Part model, mm, in its own coordinate system. A direction names the side the tool comes from. Round coordinates to 2 decimals unless told otherwise and drop trailing zeros. Loops run counter-clockwise (first coordinate to the right, second up) from the corner with the lowest first, then second, coordinate; pieces in that order, holes last. Notation, with made-up numbers: M 78,11 L 118,11 A31 ccw 118,49 Z; hole C 36.5,28 d6. An arc over 180 degrees is marked long. Answer as CSV lines item,"result". Start each with the question number.
Item 1: Wall check: line 1 (X direction, y = 2.6, z = -37); line 2 (X direction, y = 1.75, z = -47.5); line 3 (X direction, y = 0.7, z = -57). Give the ranges that are in metal, low to high.
Item 2: Drop a flat-ended pin along its axis: pin 1 Ø1 at (x, y) = (46.5, 2.5) entering from -Z. Give the stop position or say it passes through.
Item 3: Which spindle directions (+Z, -Z, +X, -X, +Y, -Y) get a long thin tool onto all of the face, cutting with end or side? Do faces 1 (the flat face through (44.723, 1, -36)), 2 (the flat face through (49, 1, 0)), 3 (the flat face through (11, 1, -55.08)). Say none if no direction does.
Item 4: Band-saw the part on B-B (y = 2.45). Give the cut face in (x, z), and give its area (3 significant figures).
Item 5: Band-saw the part on C-C (x = 59). Give the cut face in (y, z).
Item 6: Band-saw the part on D-D (x = 15.5). Give the cut face in (y, z).
Item 7: Band-saw the part on A-A (z = -29.5). Give the cut face in (x, y), and give its area (3 significant figures).
```python
from build123d import *

# Parameters (mm, degrees)
BOSS_EXTRUDE1_DEPTH = 2.9
SKETCH2_W           = 15.24
SKETCH2_H           = 1.45
CUT_EXTRUDE1_DEPTH  = 1.45
FILLET2_R           = 2.54


with BuildPart() as part:
    # Sketch1 → Boss-Extrude1 (new body)
    with BuildSketch(Plane(origin=(0, 0, 0), x_dir=(1, 0, 0), z_dir=(0, 1, 0))):
        Polygon((0, 0), (0, 55.080000076), (22.080000036, 55.080000076), (22.080000036, 44.32387376), (44.723008852, 44.32387376), (44.723008852, 27.937097796), (63.88136576, 27.937097796), (63.88136576, 71.117097796), (97.207622704, 71.117097796), (97.207622704, 0), align=None)
    extrude(amount=BOSS_EXTRUDE1_DEPTH)

    # Sketch2 → Cut-Extrude1 (cut)
    with BuildSketch(Plane(origin=(0, 0, -27.937097796), x_dir=(-1, 0, 0), z_dir=(0, 0, -1))):
        with Locations((-54.302187306, 0.725)):
            Rectangle(SKETCH2_W, SKETCH2_H)
    extrude(amount=-CUT_EXTRUDE1_DEPTH, mode=Mode.SUBTRACT)

    # Fillet2
    # the kernel refuses this fillet: 2.54 mm, written as the material it adds along each edge
    with BuildSketch(Plane(origin=(65.547187306, 1.45, -26.487097796), x_dir=(0, -1, 0), z_dir=(-1, 0, 0))) as fillet2_piece_1:
        with BuildLine():
            CenterArc((2.368220922, -2.368220922), FILLET2_R, 111.192609021, 47.614781958)
            Line((0, -1.45), (0, 0))
            Line((0, 0), (1.45, 0))
        make_face()
    extrude(amount=22.49)


solid = part.part
```
Answer block:
1,line 1,"x = 0 to 44.72, 63.88 to 97.21"
1,line 2,"x = 0 to 22.08, 63.88 to 97.21"
1,line 3,"x = 63.88 to 97.21"
2,pin 1,"stops at z = -27.94"
3,face 1,"-Z, +Y, -Y"
3,face 2,"+Z, +X, -X, +Y, -Y"
3,face 3,"-Z, -X, +Y, -Y"
4,outline,"M 0,-55.08 L 22.08,-55.08 L 22.08,-44.32 L 44.72,-44.32 L 44.72,-27.94 L 63.88,-27.94 L 63.88,-71.12 L 97.21,-71.12 L 97.21,0 L 0,0 Z"
4,area,"5,130 mm^2"
5,outline,"M 0,-26.49 A2.54 cw 1.45,-27.94 L 2.9,-27.94 L 2.9,0 L 0,0 Z"
6,outline,"M 0,-55.08 L 2.9,-55.08 L 2.9,0 L 0,0 Z"
7,outline,"M 0,0 L 44.72,0 L 44.72,2.9 L 0,2.9 Z; M 63.88,0 L 97.21,0 L 97.21,2.9 L 63.88,2.9 Z"
7,area,"226 mm^2"
